from build123d import *

# Parameters (mm, degrees)
SKETCH1_R           = 1.5
BOSS_EXTRUDE1_DEPTH = 39
FILLET1_R           = 1


with BuildPart() as part:
    # Sketch1 → Boss-Extrude1 (new body)
    with BuildSketch(Plane.XY):
        with BuildLine():
            Line((40.05, 7.5), (0, 7.5))
            ThreePointArc((0, 7.5), (-7.5, 0), (0, -7.5))
            Line((0, -7.5), (42, -7.5))
            Line((42, -7.5), (48.530525776, 3.688120536))
            ThreePointArc((48.530525776, 3.688120536), (45.780813139, 6.477302835), (42, 7.5))
            Line((42, 7.5), (40.05, 7.5))
        make_face()
        Circle(SKETCH1_R, mode=Mode.SUBTRACT)
        with Locations((42, 0)):
            Circle(SKETCH1_R, mode=Mode.SUBTRACT)
        with BuildLine():
            Line((71.033420644, 20.238824327), (40.05, 7.5))
            Line((40.05, 7.5), (42, 7.5))
            ThreePointArc((42, 7.5), (45.780813139, 6.477302835), (48.530525776, 3.688120536))
            Line((48.530525776, 3.688120536), (60.929817382, 10.690632061))
            Line((60.929817382, 10.690632061), (77.239530905, 6.459175571))
            Line((77.239530905, 6.459175571), (78.403975083, 6.2567657))
            Line((78.403975083, 6.2567657), (79.089287361, 7.219702396))
            Line((79.089287361, 7.219702396), (80.253731539, 7.017292525))
            Line((80.253731539, 7.017292525), (80.939043817, 7.980229222))
            Line((80.939043817, 7.980229222), (82.103487996, 7.777819351))
            Line((82.103487996, 7.777819351), (82.788800274, 8.740756047))
            Line((82.788800274, 8.740756047), (83.953244452, 8.538346176))
            Line((83.953244452, 8.538346176), (84.63855673, 9.501282873))
            Line((84.63855673, 9.501282873), (85.803000908, 9.298873002))
            Line((85.803000908, 9.298873002), (86.488313186, 10.261809698))
            Line((86.488313186, 10.261809698), (84.777127829, 14.423761725))
            Line((84.777127829, 14.423761725), (71.033420644, 20.238824327))
        make_face()
    extrude(amount=BOSS_EXTRUDE1_DEPTH)

    # Fillet1
    fillet1_edges = [part.edges().sort_by_distance(p)[0] for p in [
        (42, -7.5, 19.5),
        (40.05, 7.5, 19.5),
        (71.033420644, 20.238824327, 19.5),
        (84.777127829, 14.423761725, 19.5),
        (86.488313186, 10.261809698, 19.5),
        (77.239530905, 6.459175571, 19.5),
        (60.929817382, 10.690632061, 19.5),
        (48.530525776, 3.688120536, 19.5),
    ]]
    fillet(fillet1_edges, radius=FILLET1_R)


solid = part.part
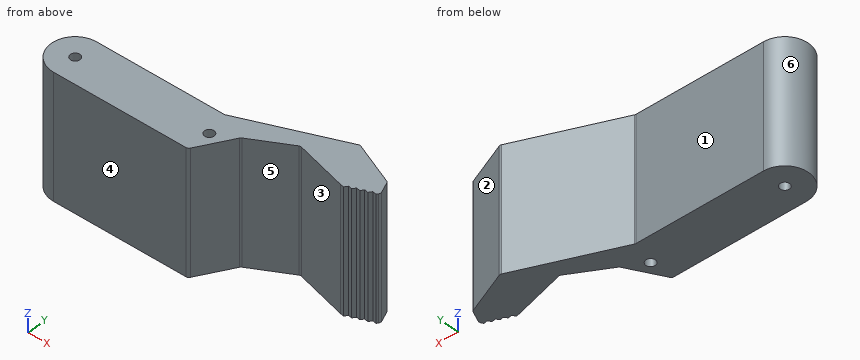
Here's how the part is built. I have some questions about the finished solid (model axes, mm). Face numbers are marked on the shaded views. A direction names the side the tool comes from. Give positions to 0.01 mm unless a question says otherwise; leave off trailing zeros. Order: outer loops, then holes, each group sorted by start corner. A loop starts at its lowest first (then second) coordinate and runs counter-clockwise, first axis right, second up. Notation, with made-up numbers: (4, -20) -> (61, -20) arc R20 ccw to (61, 4) -> close; hole circle Ø6 at (6, 89). An arc over 180 degrees is marked (long way). One line per item, written item: value. Start each with the question number.
1. For the marked faces 1 and 2, which set-ups out of +Z, -Z, +X, -X, +Y, -Y let a thin tool reach every point of the face, with its end or its side?
2. Will these pins go through, and if not, where does the flat tip stop? pin 1 Ø6 at (x, y) = (48, 8) entering from -Z; pin 2 Ø2 at (y, z) = (-1.5, 24.5) entering from +X; pin 3 Ø4 at (x, z) = (42, 35) entering from +Y; pin 4 Ø3 at (x, z) = (57.5, 32.5) entering from +Y.
3. Imagine slicing it at D-D, the plane y = 5.25. List the corners of the cut face in (x, z) for me, plus the area to 3 significant figures.
4. Imagine slicing it at A-A, the plane z = 29. List the corners of the cut face in (x, y) for me, plus the area to 3 significant figures.
5. I need wall thicknesses on probe 1 along Y at (x, z) = (0, 28); probe 2 along Y at (x, z) = (19, 22.5); probe 3 along Y at (x, z) = (42, 23). Which ranges of each line are inside material? Lowest first, please. Write a range as from..to.
6. Imagine slicing it at C-C, the plane x = 32.5. List the corners of the cut face in (y, z) for me, plus the area to 3 significant figures.
7. Imagine slicing it at B-B, the plane y = 0. List the corners of the cut face in (x, z) for me.
8. We'd pull the mould along X, two halves only. Please class the marked faces 3, 4, 5 and 6: released by +X, released by -X, zero draft, split by the parting line, or undercut.
Values follow:
1. face 1: +Z, -Z, -X, +Y
1. face 2: +Z, -Z, +X, +Y
2. pin 1: stops at z = 0
2. pin 2: stops at x = 46.09
2. pin 3: stops at y = 9.12
2. pin 4: stops at y = 15.29
3. outline: (-5.36, 0) -> (51.3, 0) -> (51.3, 39) -> (-5.36, 39) -> close
3. area: 2,210 mm2
4. outline: (0, -7.5) -> (41.43, -7.5) arc R1 ccw to (42.29, -7) -> (48.39, 3.45) arc R1 cw to (48.77, 3.82) -> (60.58, 10.49) arc R1 cw to (61.32, 10.59) -> (77.24, 6.46) -> (78.4, 6.26) -> (79.09, 7.22) -> (80.25, 7.02) -> (80.94, 7.98) -> (82.1, 7.78) -> (82.79, 8.74) -> (83.95, 8.54) -> (84.64, 9.5) -> (85.8, 9.3) -> (86.17, 9.81) arc R1 ccw to (86.28, 10.77) -> (84.93, 14.04) arc R1 ccw to (84.4, 14.58) -> (71.42, 20.08) arc R1 ccw to (70.65, 20.08) -> (40.23, 7.58) arc R1 cw to (39.85, 7.5) -> (0, 7.5) arc R7.5 ccw to start; hole circle Ø3 at (0, 0); hole circle Ø3 at (42, 0)
4. area: 1,090 mm2
5. probe 1: y = -7.5..-1.5, 1.5..7.5
5. probe 2: y = -7.5..7.5
5. probe 3: y = -7.32..-1.5, 1.5..8.3
6. outline: (-7.5, 0) -> (7.5, 0) -> (7.5, 39) -> (-7.5, 39) -> close
6. area: 585 mm2
7. outline: (-7.5, 0) -> (-1.5, 0) -> (-1.5, 39) -> (-7.5, 39) -> close; (1.5, 0) -> (40.5, 0) -> (40.5, 39) -> (1.5, 39) -> close; (43.5, 0) -> (46.38, 0) -> (46.38, 39) -> (43.5, 39) -> close
8. face 3: undercut
8. face 4: zero draft
8. face 5: undercut
8. face 6: released by -X
